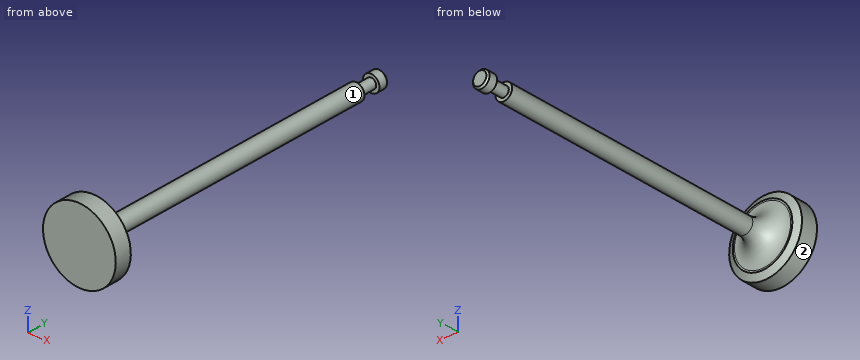
```python
from build123d import *

# Parameters (mm, degrees)
FILLET1_R      = 6
CHAMFER1_SIZE  = 1
CHAMFER1_SIZE2 = 2
CHAMFER3_SIZE  = 0.5


with BuildPart() as part:
    # Sketch1 → Revolve1 (revolve)
    with BuildSketch(Plane(origin=(0, 0, 0), x_dir=(0, 0, -1), z_dir=(1, 0, 0))):
        Polygon((0, 0), (0, -100), (11, -100), (11, -94), (2.5, -94), (2.5, -8), (1.5, -8), (1.5, -3), (2.5, -3), (2.5, 0), align=None)
    revolve(axis=Axis((0, 0, 0), (0, -1, 0)))

    # Fillet1
    fillet1_edges = [part.edges().sort_by_distance(p)[0] for p in [
        (0, -94, 2.5),
    ]]
    fillet(fillet1_edges, radius=FILLET1_R)

    # Chamfer1
    chamfer1_edges = [part.edges().sort_by_distance(p)[0] for p in [
        (0, -94, 11),
    ]]
    chamfer1_side = [part.faces().sort_by_distance(p)[0] for p in [
        (0, -97, 11),
    ]]
    chamfer(chamfer1_edges, length=CHAMFER1_SIZE, length2=CHAMFER1_SIZE2, reference=chamfer1_side[0])

    # Chamfer3
    chamfer3_edges = [part.edges().sort_by_distance(p)[0] for p in [
        (0, 0, 2.5),
    ]]
    chamfer(chamfer3_edges, length=CHAMFER3_SIZE)


solid = part.part
```
The model under review builds one solid part; all positions refer to its coordinate system, in mm. Face numbers are marked on the shaded views. A direction names the side the tool comes from. Round coordinates to 2 decimals unless told otherwise and drop trailing zeros. Loops run counter-clockwise (first coordinate to the right, second up) from the corner with the lowest first, then second, coordinate; pieces in that order, holes last.
1) Consider section D-D on y = -93. State the section outline as (x, z) points.
Values follow:
outline: circle Ø10.37 at (0, 0)
2) Tool access review of the marked faces 1 and 2: name each direction out of +Z, -Z, +X, -X, +Y, -Y from which nothing blocks a thin tool from reaching the whole face with its end or side.
Values follow:
face 1: +Y
face 2: +Y, -Y
3) Consider section A-A on z = 0. State the section outline as (x, y) points, then the cut area to 3 significant figures.
Values follow:
outline: (-11, -100) - (11, -100) - (11, -95) - (9, -94) - (8.5, -94) arc R6 cw to (2.5, -88) - (2.5, -8) - (1.5, -8) - (1.5, -3) - (2.5, -3) - (2.5, -0.5) - (2, 0) - (-2, 0) - (-2.5, -0.5) - (-2.5, -3) - (-1.5, -3) - (-1.5, -8) - (-2.5, -8) - (-2.5, -88) arc R6 cw to (-8.5, -94) - (-9, -94) - (-11, -95) - close
area: 605 mm2
4) Consider section C-C on y = -36. State the section outline as (x, z) points.
Values follow:
outline: circle Ø5 at (0, 0)
5) Consider section B-B on x = 0. State the section outline as (y, z) points.
Values follow:
outline: (-100, -11) - (-95, -11) - (-94, -9) - (-94, -8.5) arc R6 cw to (-88, -2.5) - (-8, -2.5) - (-8, -1.5) - (-3, -1.5) - (-3, -2.5) - (-0.5, -2.5) - (0, -2) - (0, 2) - (-0.5, 2.5) - (-3, 2.5) - (-3, 1.5) - (-8, 1.5) - (-8, 2.5) - (-88, 2.5) arc R6 cw to (-94, 8.5) - (-94, 9) - (-95, 11) - (-100, 11) - close
6) Wall thickness on line 1 along Z through (x, y) = (2, -86); line 2 along X through (y, z) = (-15, 0); line 3 along X through (y, z) = (-57, 1.5): over which ranges is each line inside the solid? List them lowest first.
Values follow:
line 1: z = -1.5 to 1.5
line 2: x = -2.5 to 2.5
line 3: x = -2 to 2
7) Clearance check with flat-ended pins moving along their axes: P1, Ø2, axis at y = -24, z = 2.5, coming from the +X side; P2, Ø5, axis at x = 6.5, y = -44.5, coming from the -Z side; P3, Ø10, axis at x = 0.5, y = -16, coming from the +Z side; P4, Ø4, axis at x = 0, y = -47, coming from the -Z side. State where each tip first meets the part, or that it passes through.
Values follow:
P1: stops at x = 2
P2: passes through
P3: stops at z = 2.5
P4: stops at z = -2.5
